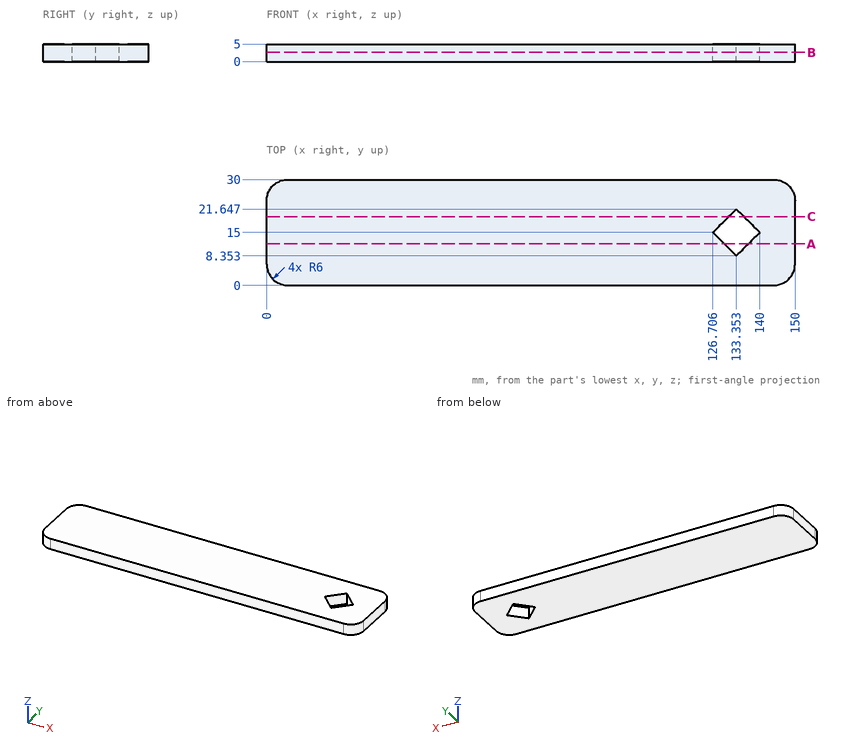
Part print with two shaded views. Sizes in mm from the minimum x, y, z corner. Coordinates: 2 decimals unless noted, no trailing zeros. Write each loop counter-clockwise with the first axis right and the second up, starting at its lowest first coordinate (ties: lowest second). Pieces come first, ordered by that corner, then holes. Notation, with made-up numbers: (-2.5, 34.5) -> (3.5, 34.5) arc R16 cw to (3.5, 46.5) -> close; hole circle Ø4 at (51.5, 51). An arc over 180 degrees is marked (long way). Return JSON: item names as keys, results as strings. Group by question number.
Q1. Drill centre lines: line 1 (Y direction, x = 132.5, z = 1.25) (1 decimal); line 2 (Y direction, x = 135.5, z = 2.1); line 3 (X direction, y = 27.75, z = 2.3) (1 decimal). Where is each one in solid material? Low to high.
Q2. Cut at C-C, the plane y = 19.5. Give the cut face in (x, z).
Q3. Cut at B-B, the plane z = 2.6. Give the cut face in (x, y), then the cut area to 3 significant figures.
Q4. Cut at A-A, the plane y = 11.75. Give the cut face in (x, z).
Returned:
{
 "1": {"line 1": "y = 0 to 9.2, 20.8 to 30", "line 2": "y = 0 to 10.5, 19.5 to 30", "line 3": "x = 1.3 to 148.7"},
 "2": {"outline": "(0, 0) -> (131.21, 0) -> (131.21, 5) -> (0, 5) -> close; (135.5, 0) -> (150, 0) -> (150, 5) -> (135.5, 5) -> close"},
 "3": {"outline": "(0, 6) arc R6 ccw to (6, 0) -> (144, 0) arc R6 ccw to (150, 6) -> (150, 24) arc R6 ccw to (144, 30) -> (6, 30) arc R6 ccw to (0, 24) -> close; hole (126.71, 15) -> (133.35, 8.35) -> (140, 15) -> (133.35, 21.65) -> close", "area": "4,380 mm2"},
 "4": {"outline": "(0, 0) -> (129.96, 0) -> (129.96, 5) -> (0, 5) -> close; (136.75, 0) -> (150, 0) -> (150, 5) -> (136.75, 5) -> close"}
}
